Autodesk Inventor part; units mm, degrees
ref_plane "YZ Plane" through (0, 0, 0) normal (1, 0, 0) x (0, 1, 0)
ref_plane "XZ Plane" through (0, 0, 0) normal (0, 1, 0) x (-1, 0, 0)
ref_plane "XY Plane" through (0, 0, 0) normal (0, 0, 1) x (1, 0, 0)
sketch "Sketch1" plane through (0, 0, 0) normal (0, 0, 1) x (1, 0, 0)
  circle A0 centre (0, 0) radius 15.875
  line L0 (3.6662, 6.35) -> (7.3323, 0)
  line L1 (7.3323, 0) -> (3.6662, -6.35)
  line L2 (3.6662, -6.35) -> (-3.6662, -6.35)
  line L3 (-3.6662, -6.35) -> (-7.3323, 0)
  line L4 (-7.3323, 0) -> (-3.6662, 6.35)
  line L5 (-3.6662, 6.35) -> (3.6662, 6.35)
  dimension "d0" = 31.75
  dimension "d1" = 12.7
extrude "Extrusion1" add sketch "Sketch1" along normal blind 7.9248
sketch "Sketch2" plane through (0, 0, 7.9248) normal (0, 0, 1) x (1, 0, 0)
  circle A0 centre (0, 0) radius 15.875
  circle A1 centre (0, 0) radius 15.875
  circle A2 centre (0, 0) radius 14.2875
  dimension "d4" = 1.5875
extrude "Extrusion2" cut sketch "Sketch2" against normal blind 6.3373
properties part number "500id_1.125od_hex_flange_bearing" material "Stainless Steel, 440C"
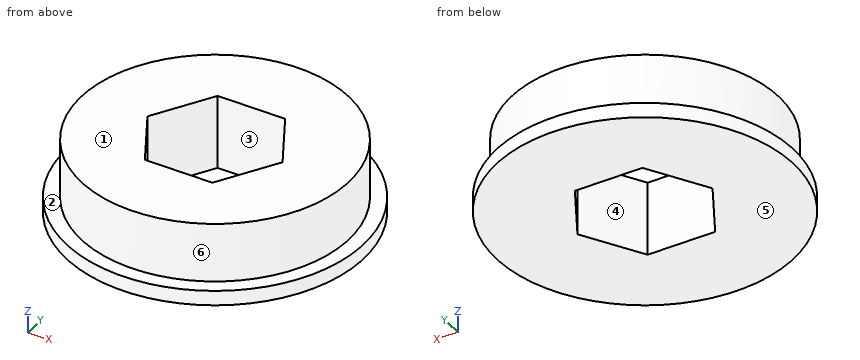
Verification items for the finished model (mm, model axes). Face numbers are marked on the shaded views. A direction names the side the tool comes from. Round coordinates to 2 decimals unless told otherwise and drop trailing zeros. Order: outer loops, then holes, each group sorted by start corner. A loop starts at its lowest first (then second) coordinate and runs counter-clockwise, first axis right, second up.
1. Section check B-B on y = -3. Record the cut outline in (x, z), then the cut area to 3 significant figures.
Final values:
outline: (-15.59, 0) - (-5.6, 0) - (-5.6, 7.92) - (-13.97, 7.92) - (-13.97, 1.59) - (-15.59, 1.59) - close; (5.6, 0) - (15.59, 0) - (15.59, 1.59) - (13.97, 1.59) - (13.97, 7.92) - (5.6, 7.92) - close
area: 138 mm2
2. Go/stop test with flat-tipped pins: P1, Ø2, axis at y = -11, z = 4.5, coming from the -X side; P2, Ø3, axis at y = -11, z = 3.5, coming from the -X side; P3, Ø3, axis at x = 8, z = 7, coming from the -Y side. Record where each tip stops, or that it passes through.
Final values:
P1: stops at x = -10.2
P2: stops at x = -10.67
P3: stops at y = -12.72
3. Access from +Z, -Z, +X, -X, +Y, -Y to the whole of each face (thin tool, end or side, straight path). Record for the marked faces 1, 2 and 3.
Final values:
face 1: +Z, +X, -X, +Y, -Y
face 2: +Z
face 3: +Z, -Z
4. Release check for a two-part mould opening along Y. For the marked faces 4, 5 and 6 record: +Y half, -Y half, draft (parallel to the pull), parting line (faces both ways), or undercut.
Final values:
face 4: undercut
face 5: draft
face 6: parting line
5. Section check C-C on z = 1. Record the cut outline in (x, y) (3 decimals), then the cut area to 3 significant figures.
Final values:
outline: circle Ø31.75 at (0, 0); hole (-7.332, 0) - (-3.666, -6.35) - (3.666, -6.35) - (7.332, 0) - (3.666, 6.35) - (-3.666, 6.35) - close
area: 652 mm2
6. Thickness scan on L1, parallel to Y at x = -3, z = 5.5; L2, parallel to X at y = -1, z = 1.5; L3, parallel to X at y = -1.5, z = 5. Record the ranges inside material, lowest first.
Final values:
L1: y = -13.97 to -6.35, 6.35 to 13.97
L2: x = -15.84 to -6.75, 6.75 to 15.84
L3: x = -14.21 to -6.47, 6.47 to 14.21
